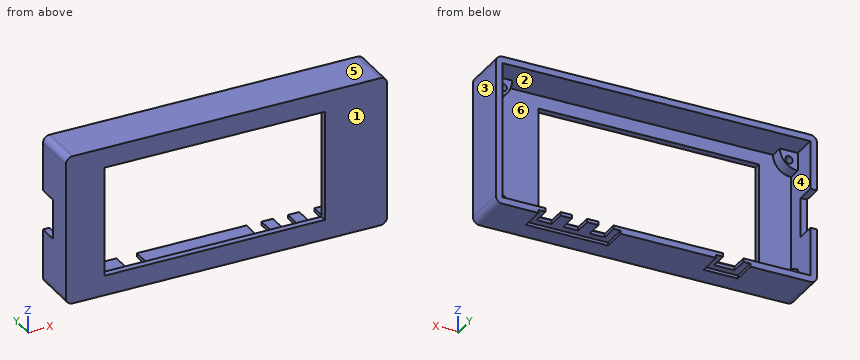
from build123d import *

# Parameters (mm, degrees)
SKETCH_1_W          = 69.855
SKETCH_1_H          = 30.988
EXTRUDE_1_DEPTH     = 1.5
CUT_EXTRUDE_2_REACH = 3.5
SKETCH_1_6_W        = 50
SKETCH_1_6_H        = 24.956
SKETCH_1_7_W        = 72.855
SKETCH_1_7_H        = 33.988
SKETCH_1_7_W_2      = 69.855
SKETCH_1_7_H_2      = 30.988
EXTRUDE_1_2_DEPTH   = 10
FILLET_1_R          = 1.5
EXTRUDE_2_DEPTH     = 3
CUT_EXTRUDE_3_REACH = 3.5
SKETCH_4_W          = 9
SKETCH_4_H          = 4.3
CUT_EXTRUDE_4_REACH = 3.5
SKETCH_5_W          = 3.4
SKETCH_5_H          = 4
SKETCH_5_W_2        = 4.6
CUT_EXTRUDE_START   = -1.5
SKETCH_5_6_W        = 7.8
SKETCH_5_6_H        = 7.2
SKETCH_5_6_W_2      = 18.6
CUT_EXTRUDE_6_DEPTH = 0.7
SKETCH_3_R          = 0.85
CUT_EXTRUDE_7_DEPTH = 3


with BuildPart() as part:
    # Sketch 1 → Extrude 1 (new body)
    with BuildSketch(Plane(origin=(0, 0, 0), x_dir=(1, 0, 0), z_dir=(0, 1, 0))):
        Rectangle(SKETCH_1_W, SKETCH_1_H)
    extrude(amount=EXTRUDE_1_DEPTH)

    # Sketch 1_6 → Cut-Extrude 2 (cut, up to next)
    with BuildSketch(Plane(origin=(0, 0, 0), x_dir=(1, 0, 0), z_dir=(0, 1, 0)), mode=Mode.PRIVATE) as cut_extrude_2_sk1:
        with Locations((-2.6635, 0)):
            Rectangle(SKETCH_1_6_W, SKETCH_1_6_H)
    cut_extrude_2_tool1 = extrude(cut_extrude_2_sk1.sketch, amount=CUT_EXTRUDE_2_REACH, mode=Mode.PRIVATE) & part.part
    add(cut_extrude_2_tool1.solids().sort_by_distance((-2.6635, 0, 0))[0], mode=Mode.SUBTRACT)



with BuildPart() as body_2:
    # Sketch 1_7 → Extrude 1 2 (new body)
    with BuildSketch(Plane(origin=(0, 0, 0), x_dir=(1, 0, 0), z_dir=(0, 1, 0))):
        Rectangle(SKETCH_1_7_W, SKETCH_1_7_H)
        Rectangle(SKETCH_1_7_W_2, SKETCH_1_7_H_2, mode=Mode.SUBTRACT)
    extrude(amount=EXTRUDE_1_2_DEPTH)

    # Fillet 1
    fillet_1_edges = [body_2.edges().sort_by_distance(p)[0] for p in [
        (-36.4275, 5, -16.994),
        (-36.4275, 5, 16.994),
        (36.4275, 5, 16.994),
        (36.4275, 5, -16.994),
    ]]
    fillet(fillet_1_edges, radius=FILLET_1_R)


with BuildPart() as part_1:
    add(part.part)

    add(body_2.part)  # Extrude 2 merges body 2
    # Sketch 2 → Extrude 2 (add)
    with BuildSketch(Plane(origin=(0, 1.5, 0), x_dir=(1, 0, 0), z_dir=(0, 1, 0))):
        with BuildLine():
            ThreePointArc((-30.8635, -15.494), (-32.053818041, -12.620318041), (-34.9275, -11.43))
            Line((-34.9275, -11.43), (-34.9275, -15.494))
            Line((-34.9275, -15.494), (-30.8635, -15.494))
        make_face()
        with BuildLine():
            ThreePointArc((-34.9275, 11.43), (-32.053818041, 12.620318041), (-30.8635, 15.494))
            Line((-30.8635, 15.494), (-34.9275, 15.494))
            Line((-34.9275, 15.494), (-34.9275, 11.43))
        make_face()
        with BuildLine():
            Line((34.9275, 15.494), (29.8635, 15.494))
            ThreePointArc((29.8635, 15.494), (31.34671126, 11.91321126), (34.9275, 10.43))
            Line((34.9275, 10.43), (34.9275, 15.494))
        make_face()
        with BuildLine():
            Line((34.9275, -15.494), (34.9275, -10.43))
            ThreePointArc((34.9275, -10.43), (31.34671126, -11.91321126), (29.8635, -15.494))
            Line((29.8635, -15.494), (34.9275, -15.494))
        make_face()
    extrude(amount=EXTRUDE_2_DEPTH)

    # Sketch 4 → Cut-Extrude 3 (cut, up to next)
    with BuildSketch(Plane(origin=(-34.9275, 0, 0), x_dir=(0, 0, -1), z_dir=(1, 0, 0)), mode=Mode.PRIVATE) as cut_extrude_3_sk1:
        with Locations((0, 7.85)):
            Rectangle(SKETCH_4_W, SKETCH_4_H)
    cut_extrude_3_tool1 = extrude(cut_extrude_3_sk1.sketch, amount=-CUT_EXTRUDE_3_REACH, mode=Mode.PRIVATE) & part_1.part
    add(cut_extrude_3_tool1.solids().sort_by_distance((-34.9275, 7.85, 0))[0], mode=Mode.SUBTRACT)

    # Sketch 5 → Cut-Extrude 4 (cut, up to next)
    with BuildSketch(Plane.XY.offset(-15.494), mode=Mode.PRIVATE) as cut_extrude_4_sk1:
        with Locations((11.4275, 8.1)):
            Rectangle(SKETCH_5_W, SKETCH_5_H)
    cut_extrude_4_tool1 = extrude(cut_extrude_4_sk1.sketch, amount=-CUT_EXTRUDE_4_REACH, mode=Mode.PRIVATE) & part_1.part
    add(cut_extrude_4_tool1.solids().sort_by_distance((11.4275, 8.1, -15.494))[0], mode=Mode.SUBTRACT)
    # Sketch 5 → Cut-Extrude 4 (cut, up to next)
    with BuildSketch(Plane.XY.offset(-15.494), mode=Mode.PRIVATE) as cut_extrude_4_sk2:
        with Locations((17.4275, 8.1)):
            Rectangle(SKETCH_5_W, SKETCH_5_H)
    cut_extrude_4_tool2 = extrude(cut_extrude_4_sk2.sketch, amount=-CUT_EXTRUDE_4_REACH, mode=Mode.PRIVATE) & part_1.part
    add(cut_extrude_4_tool2.solids().sort_by_distance((17.4275, 8.1, -15.494))[0], mode=Mode.SUBTRACT)
    # Sketch 5 → Cut-Extrude 4 (cut, up to next)
    with BuildSketch(Plane.XY.offset(-15.494), mode=Mode.PRIVATE) as cut_extrude_4_sk3:
        with Locations((23.4275, 8.1)):
            Rectangle(SKETCH_5_W, SKETCH_5_H)
    cut_extrude_4_tool3 = extrude(cut_extrude_4_sk3.sketch, amount=-CUT_EXTRUDE_4_REACH, mode=Mode.PRIVATE) & part_1.part
    add(cut_extrude_4_tool3.solids().sort_by_distance((23.4275, 8.1, -15.494))[0], mode=Mode.SUBTRACT)
    # Sketch 5 → Cut-Extrude 4 (cut, up to next)
    with BuildSketch(Plane.XY.offset(-15.494), mode=Mode.PRIVATE) as cut_extrude_4_sk4:
        with Locations((-17.4275, 8.1)):
            Rectangle(SKETCH_5_W_2, SKETCH_5_H)
    cut_extrude_4_tool4 = extrude(cut_extrude_4_sk4.sketch, amount=-CUT_EXTRUDE_4_REACH, mode=Mode.PRIVATE) & part_1.part
    add(cut_extrude_4_tool4.solids().sort_by_distance((-17.4275, 8.1, -15.494))[0], mode=Mode.SUBTRACT)

    # Sketch 5_6 → Cut-Extrude 6 (cut)
    with BuildSketch(Plane.XY.offset(-15.494).offset(CUT_EXTRUDE_START)):
        with Locations((-17.4275, 8.1)):
            Rectangle(SKETCH_5_6_W, SKETCH_5_6_H)
        with Locations((17.4275, 8.1)):
            Rectangle(SKETCH_5_6_W_2, SKETCH_5_6_H)
    extrude(amount=CUT_EXTRUDE_6_DEPTH, mode=Mode.SUBTRACT)

    # Sketch 3 → Cut-Extrude 7 (cut)
    with BuildSketch(Plane(origin=(0, 4.5, 0), x_dir=(1, 0, 0), z_dir=(0, 1, 0))):
        with Locations((-32.9275, -13.394)):
            Circle(SKETCH_3_R)
        with Locations((-32.9275, 13.394)):
            Circle(SKETCH_3_R)
        with Locations((31.9275, -13.394)):
            Circle(SKETCH_3_R)
        with Locations((31.9275, 13.394)):
            Circle(SKETCH_3_R)
    extrude(amount=-CUT_EXTRUDE_7_DEPTH, mode=Mode.SUBTRACT)


solid = part_1.part
Read the model definition and answer for the solid it produces. Units are mm, in the model's axes. Face numbers are marked on the shaded views. A direction names the side the tool comes from. Round coordinates to 2 decimals unless told otherwise and drop trailing zeros. Order: outer loops, then holes, each group sorted by start corner. A loop starts at its lowest first (then second) coordinate and runs counter-clockwise, first axis right, second up.
1) For the marked faces 5 and 6, determine the directions among +Z, -Z, +X, -X, +Y, -Y from which every point of the face is accessible in a straight line to the end or side of a thin tool.
2) The mould has two halves that part along X. Classify the marked faces 1, 2, 3 and 4: released by +X, released by -X, zero draft, split by the parting line, or undercut.
3) The part is cut by section B-B on x = 5.5. Write down the section's boundary in (y, z).
4) Straight lines are drawn through the part: L1, parallel to X at y = 3, z = 3.5; L2, parallel to Z at x = -11.5, y = 6.75; L3, parallel to Z at x = -17, y = 5. For each, find the intervals that lie inside material, in ascending order.
5) Flat-ended cylindrical pins translate along their axes: pin 1 (0.6 mm diameter, centred on x = 12, z = -16, fed in from +Y); pin 2 (1.2 mm diameter, centred on x = -35.5, z = -1.5, fed in from +Y); pin 3 (4.5 mm diameter, centred on x = -32, z = 13, fed in from +Y). Find the tip coordinate at first contact, or state that the pin passes through.
6) The part is cut by section D-D on x = -18. Write down the section's boundary in (y, z), plus the area to 3 significant figures.
7) The part is cut by section A-A on z = 1. Write down the section's boundary in (x, y), plus the area to 3 significant figures.
8) The part is cut by section C-C on y = 9. Give the number of separate pieces and of enclosed holes in the cut face, plus the area to 3 significant figures.
Resolved:
1. face 5: +Z, +X, -X, +Y, -Y
1. face 6: +Y
2. face 1: zero draft
2. face 2: undercut
2. face 3: released by +X
2. face 4: undercut
3. outline: (0, -16.99) - (10, -16.99) - (10, -15.49) - (1.5, -15.49) - (1.5, -12.48) - (0, -12.48) - close; (0, 12.48) - (1.5, 12.48) - (1.5, 15.49) - (10, 15.49) - (10, 16.99) - (0, 16.99) - close
4. L1: x = -36.43 to -34.93, 34.93 to 36.43
4. L2: z = -16.99 to -15.49, 15.49 to 16.99
4. L3: z = -16.29 to -15.49, 15.49 to 16.99
5. pin 1: stops at y = 6.1
5. pin 2: stops at y = 5.7
5. pin 3: stops at y = 4.5
6. outline: (0, -16.99) - (4.5, -16.99) - (4.5, -16.29) - (6.1, -16.29) - (6.1, -15.49) - (1.5, -15.49) - (1.5, -12.48) - (0, -12.48) - close; (0, 12.48) - (1.5, 12.48) - (1.5, 15.49) - (10, 15.49) - (10, 16.99) - (0, 16.99) - close
6. area: 32.1 mm2
7. outline: (-36.43, 0) - (-27.66, 0) - (-27.66, 1.5) - (-34.93, 1.5) - (-34.93, 5.7) - (-36.43, 5.7) - close; (22.34, 0) - (36.43, 0) - (36.43, 10) - (34.93, 10) - (34.93, 1.5) - (22.34, 1.5) - close
7. area: 53.3 mm2
8. separate pieces: 5
8. enclosed holes: 0
8. area: 266 mm2
